Here's how the part is built. I have some questions about the finished solid (model axes, mm). Give positions to 0.01 mm unless a question says otherwise; leave off trailing zeros. Order: outer loops, then holes, each group sorted by start corner. A loop starts at its lowest first (then second) coordinate and runs counter-clockwise, first axis right, second up. Notation, with made-up numbers: M 19,27 L 45,27 A24 cw 45,40 Z; hole C 66.5,59 d4. An arc over 180 degrees is marked long. Use one line per item in the form item = value.
from build123d import *

# Parameters (mm, degrees)
SKETCH1_W           = 22.86
SKETCH1_H           = 10.16
BOSS_EXTRUDE1_DEPTH = 3.175
SKETCH2_R           = 2.5
CUT_EXTRUDE1_DEPTH  = 4.175
FILLET1_R           = 2.54


with BuildPart() as part:
    # Sketch1 → Boss-Extrude1 (new body)
    with BuildSketch(Plane(origin=(0, 0, 0), x_dir=(1, 0, 0), z_dir=(0, 1, 0))):
        Rectangle(SKETCH1_W, SKETCH1_H)
    extrude(amount=BOSS_EXTRUDE1_DEPTH)

    # Sketch2 → Cut-Extrude1 (cut, through all)
    with BuildSketch(Plane(origin=(0, 3.175, 0), x_dir=(1, 0, 0), z_dir=(0, 1, 0))):
        with Locations((-6.35, 0)):
            Circle(SKETCH2_R)
        with Locations((6.35, 0)):
            Circle(SKETCH2_R)
    extrude(amount=-CUT_EXTRUDE1_DEPTH, mode=Mode.SUBTRACT)

    # Fillet1
    fillet1_edges = [part.edges().sort_by_distance(p)[0] for p in [
        (11.43, 1.5875, 5.08),
        (-11.43, 1.5875, 5.08),
        (-11.43, 1.5875, -5.08),
        (11.43, 1.5875, -5.08),
    ]]
    fillet(fillet1_edges, radius=FILLET1_R)


solid = part.part
Q1. I want a section at A-A on x = 6.35. Write out the boundary of the cut face in (y, z) (3 decimals).
Found:
outline = M 0,-5.08 L 3.175,-5.08 L 3.175,-2.5 L 0,-2.5 Z; M 0,2.5 L 3.175,2.5 L 3.175,5.08 L 0,5.08 Z
Q2. I want a section at C-C on y = 0.6. Write out the boundary of the cut face in (x, z).
Found:
outline = M -11.43,-2.54 A2.54 ccw -8.89,-5.08 L 8.89,-5.08 A2.54 ccw 11.43,-2.54 L 11.43,2.54 A2.54 ccw 8.89,5.08 L -8.89,5.08 A2.54 ccw -11.43,2.54 Z; hole C -6.35,0 d5; hole C 6.35,0 d5
Q3. Thinking about a two-plate mould opening in X: for faces 1 (the face through (-8.334, 1.61, 1.521)), 2 (the face through (0, 2, 5.08)), 3 (the face through (-10.706, 1.61, 4.316)), 4 (the face through (3.852, 1.61, -0.11)), which applies, +X half, -X half, draft (parallel to the pull), parting line (faces both ways), or undercut?
Found:
face_1 = undercut
face_2 = draft
face_3 = -X half
face_4 = undercut
Q4. I want a section at B-B on z = 0. Write out the boundary of the cut face in (x, y) (3 decimals), then the cut area to 3 significant figures.
Found:
outline = M -11.43,0 L -8.85,0 L -8.85,3.175 L -11.43,3.175 Z; M -3.85,0 L 3.85,0 L 3.85,3.175 L -3.85,3.175 Z; M 8.85,0 L 11.43,0 L 11.43,3.175 L 8.85,3.175 Z
area = 40.8 mm²
Q5. I'm going to push a flat-ended pin straight in: pin 1 Ø4.5 at (x, z) = (6.35, 0) entering from +Y. Where does the tip first touch, or does it pass through?
Found:
pin_1 = through
Q6. I need wall thicknesses on L1, parallel to X at y = 1.1, z = 0; L2, parallel to Z at x = 6.35, y = 1.55; L3, parallel to X at y = 1.3, z = 1.5. Which ranges of each line are inside material? Lowest first, please.
Found:
L1 = -11.43 to -8.85, -3.85 to 3.85, 8.85 to 11.43
L2 = -5.08 to -2.5, 2.5 to 5.08
L3 = -11.43 to -8.35, -4.35 to 4.35, 8.35 to 11.43
Q7. I want a section at D-D on z = -1.75. Write out the boundary of the cut face in (x, y) (3 decimals), then the cut area to 3 significant figures.
Found:
outline = M -11.43,0 L -8.135,0 L -8.135,3.175 L -11.43,3.175 Z; M -4.565,0 L 4.565,0 L 4.565,3.175 L -4.565,3.175 Z; M 8.135,0 L 11.43,0 L 11.43,3.175 L 8.135,3.175 Z
area = 49.9 mm²
